Could you check a few things on this model? Use its own coordinates, in mm. A direction names the side the tool comes from. Round coordinates to 2 decimals unless told otherwise and drop trailing zeros. Loops run counter-clockwise (first coordinate to the right, second up) from the corner with the lowest first, then second, coordinate; pieces in that order, holes last. Notation, with made-up numbers: (-12.5, 62) - (34.5, 62) arc R28 cw to (34.5, 100) - close; hole circle Ø9 at (79, -28.75). An arc over 180 degrees is marked (long way). Use one line per item in the form item = value.
```python
from build123d import *

# Parameters (mm, degrees)
SKETCH1_W                = 200
SKETCH1_H                = 200
SKETCH1_R                = 5
BOSS_EXTRUDE1_DEPTH      = 10
SKETCH2_W                = 30
SKETCH2_H                = 5
CUT_EXTRUDE1_DEPTH       = 5
BOSS_EXTRUDE3_START      = 5
BOSS_EXTRUDE3_DEPTH      = 5
CIRPATTERN1_COUNT        = 4
CIRPATTERN1_START        = 5
CIRPATTERN1_COPY_1_DEPTH = 5
CIRPATTERN1_COPY_2_DEPTH = 5
CIRPATTERN1_COPY_3_DEPTH = 5


with BuildPart() as part:
    # Sketch1 → Boss-Extrude1 (new body)
    with BuildSketch(Plane(origin=(0, 0, 0), x_dir=(1, 0, 0), z_dir=(0, 1, 0))):
        Rectangle(SKETCH1_W, SKETCH1_H)
        with Locations(Location((0, 0, 0), (0, 0, 270))):
            Circle(SKETCH1_R, mode=Mode.SUBTRACT)
    extrude(amount=BOSS_EXTRUDE1_DEPTH)

    # Sketch2 → Cut-Extrude1 (cut)
    with BuildSketch(Plane(origin=(0, 10, 0), x_dir=(1, 0, 0), z_dir=(0, 1, 0))):
        with Locations((45, 97.5)):
            Rectangle(SKETCH2_W, SKETCH2_H)
        with Locations((-45, 97.5)):
            Rectangle(SKETCH2_W, SKETCH2_H)
    cut_extrude1 = extrude(amount=-CUT_EXTRUDE1_DEPTH, mode=Mode.SUBTRACT)

    # Sketch3 → Boss-Extrude3 (add)
    with BuildSketch(Plane.ZY.offset(-60).offset(BOSS_EXTRUDE3_START)):
        with BuildLine():
            Line((-97.5, 10), (-95, 10))
            ThreePointArc((-95, 10), (-103.535533906, 13.535533906), (-100, 5))
            Line((-100, 5), (-100, 7.5))
            ThreePointArc((-100, 7.5), (-101.767766953, 11.767766953), (-97.5, 10))
        make_face()
        with BuildLine():
            ThreePointArc((-100, 5), (-96.464466094, 6.464466094), (-95, 10))
            Line((-95, 10), (-97.5, 10))
            ThreePointArc((-97.5, 10), (-98.232233047, 8.232233047), (-100, 7.5))
            Line((-100, 7.5), (-100, 5))
        make_face()
        with BuildLine():
            Line((-95, 5), (-95, 10))
            ThreePointArc((-95, 10), (-96.464466094, 6.464466094), (-100, 5))
            Line((-100, 5), (-95, 5))
        make_face()
    boss_extrude3 = extrude(amount=BOSS_EXTRUDE3_DEPTH)

    # Mirror1: Boss-Extrude3 across plane
    add(boss_extrude3.mirror(Plane(origin=(0, 0, 0), x_dir=(0, 0, 1), z_dir=(1, 0, 0))))

    # CirPattern1: Cut-Extrude1, Boss-Extrude3 ×4 about axis
    cirpattern1_axis = Axis((0, 0, 0), (0, 1, 0))
    add([cut_extrude1.rotate(cirpattern1_axis, i * 360 / CIRPATTERN1_COUNT) for i in range(1, CIRPATTERN1_COUNT)], mode=Mode.SUBTRACT)
    add([boss_extrude3.rotate(cirpattern1_axis, i * 360 / CIRPATTERN1_COUNT) for i in range(1, CIRPATTERN1_COUNT)])

    # CirPattern1 copy 1 sketch → CirPattern1 copy 1 (add)
    with BuildSketch(Plane(origin=(0, 0, 60), x_dir=(1, 0, 0), z_dir=(0, 0, -1)).offset(CIRPATTERN1_START)):
        with BuildLine():
            Line((-97.5, -10), (-95, -10))
            ThreePointArc((-95, -10), (-103.535533906, -13.535533906), (-100, -5))
            Line((-100, -5), (-100, -7.5))
            ThreePointArc((-100, -7.5), (-101.767766953, -11.767766953), (-97.5, -10))
        make_face()
        with BuildLine():
            ThreePointArc((-100, -5), (-96.464466094, -6.464466094), (-95, -10))
            Line((-95, -10), (-97.5, -10))
            ThreePointArc((-97.5, -10), (-98.232233047, -8.232233047), (-100, -7.5))
            Line((-100, -7.5), (-100, -5))
        make_face()
        with BuildLine():
            Line((-95, -5), (-95, -10))
            ThreePointArc((-95, -10), (-96.464466094, -6.464466094), (-100, -5))
            Line((-100, -5), (-95, -5))
        make_face()
    extrude(amount=CIRPATTERN1_COPY_1_DEPTH)

    # CirPattern1 copy 2 sketch → CirPattern1 copy 2 (add)
    with BuildSketch(Plane(origin=(60, 0, 0), x_dir=(0, 0, -1), z_dir=(-1, 0, 0)).offset(CIRPATTERN1_START)):
        with BuildLine():
            Line((-97.5, -10), (-95, -10))
            ThreePointArc((-95, -10), (-103.535533906, -13.535533906), (-100, -5))
            Line((-100, -5), (-100, -7.5))
            ThreePointArc((-100, -7.5), (-101.767766953, -11.767766953), (-97.5, -10))
        make_face()
        with BuildLine():
            ThreePointArc((-100, -5), (-96.464466094, -6.464466094), (-95, -10))
            Line((-95, -10), (-97.5, -10))
            ThreePointArc((-97.5, -10), (-98.232233047, -8.232233047), (-100, -7.5))
            Line((-100, -7.5), (-100, -5))
        make_face()
        with BuildLine():
            Line((-95, -5), (-95, -10))
            ThreePointArc((-95, -10), (-96.464466094, -6.464466094), (-100, -5))
            Line((-100, -5), (-95, -5))
        make_face()
    extrude(amount=CIRPATTERN1_COPY_2_DEPTH)

    # CirPattern1 copy 3 sketch → CirPattern1 copy 3 (add)
    with BuildSketch(Plane(origin=(0, 0, -60), x_dir=(-1, 0, 0), z_dir=(0, 0, 1)).offset(CIRPATTERN1_START)):
        with BuildLine():
            Line((-97.5, -10), (-95, -10))
            ThreePointArc((-95, -10), (-103.535533906, -13.535533906), (-100, -5))
            Line((-100, -5), (-100, -7.5))
            ThreePointArc((-100, -7.5), (-101.767766953, -11.767766953), (-97.5, -10))
        make_face()
        with BuildLine():
            ThreePointArc((-100, -5), (-96.464466094, -6.464466094), (-95, -10))
            Line((-95, -10), (-97.5, -10))
            ThreePointArc((-97.5, -10), (-98.232233047, -8.232233047), (-100, -7.5))
            Line((-100, -7.5), (-100, -5))
        make_face()
        with BuildLine():
            Line((-95, -5), (-95, -10))
            ThreePointArc((-95, -10), (-96.464466094, -6.464466094), (-100, -5))
            Line((-100, -5), (-95, -5))
        make_face()
    extrude(amount=CIRPATTERN1_COPY_3_DEPTH)


solid = part.part
```
1. If we section it at C-C, the plane x = -77: Write out the boundary of the cut face in (y, z), plus the area to 3 significant figures.
Solution:
outline = (0, -100) - (10, -100) - (10, 100) - (0, 100) - close
area = 2,000 mm^2
2. If we section it at A-A, the plane x = 0: Write out the boundary of the cut face in (y, z).
Solution:
outline = (0, -100) - (10, -100) - (10, -5) - (0, -5) - close; (0, 5) - (10, 5) - (10, 100) - (0, 100) - close
3. Please list where these lines run through material, in increasing order: line 1 along Y through (x, z) = (-72, 26); line 2 along X through (y, z) = (5.5, 9.5); line 3 along X through (y, z) = (6, -39).
Solution:
line_1 = 0 to 10
line_2 = -100 to 100
line_3 = -95 to 95
4. If we section it at D-D, the plane z = 83: Write out the boundary of the cut face in (x, y).
Solution:
outline = (-100, 0) - (100, 0) - (100, 10) - (-100, 10) - close
5. On a 3-axis mill with a long thin cutter (end or side, diameter ignored), from which of +Z, -Z, +X, -X, +Y, -Y can I reach the whole of each face in a straight line? I mean faces 4 (the face through (-55, 8, 98)), 5 (the face through (-58, 8, -95)), 6 (the face through (-97, 8, 30)). Say none if no direction works.
Solution:
face_4 = +Z, +Y
face_5 = -Z, +Y
face_6 = -X, +Y
6. For P1, Ø1.5, axis at x = 39, y = 8.5, coming from the +Z side; P2, Ø1.5, axis at x = -97, y = 7.5, coming from the -Z side; P3, Ø3, axis at y = 4, z = 35.5, coming from the -X side, each with a flat end and sliding along its axis, tell me the tip position at first contact or that it passes through.
Solution:
P1 = 95
P2 = -100
P3 = -100
7. If we section it at B-B, the plane z = -0.5: Write out the boundary of the cut face in (x, y), plus the area to 3 significant figures.
Solution:
outline = (-100, 0) - (-4.97, 0) - (-4.97, 10) - (-100, 10) - close; (4.97, 0) - (100, 0) - (100, 10) - (4.97, 10) - close
area = 1,900 mm^2
8. We'd pull the mould along X, two halves only. Please class faces 1 (the face through (-95, 8, -40)), 2 (the face through (-40, 5, -98)), 3 (the face through (98, 8, 55)): +X half, -X half, draft (parallel to the pull), parting line (faces both ways), or undercut.
Solution:
face_1 = -X half
face_2 = undercut
face_3 = draft
